Autodesk Inventor part; units mm, degrees
ref_plane "YZ Plane" through (0, 0, 0) normal (1, 0, 0) x (0, 1, 0)
ref_plane "XZ Plane" through (0, 0, 0) normal (0, 1, 0) x (-1, 0, 0)
ref_plane "XY Plane" through (0, 0, 0) normal (0, 0, 1) x (1, 0, 0)
sketch "Sketch1" plane through (0, 0, 0) normal (0, 0, 1) x (1, 0, 0)
  circle A0 centre (0, 0) radius 6.35
  dimension "d0" = 12.7
extrude "Extrusion1" add sketch "Sketch1" along normal blind 203.2
sketch "Sketch5" plane through (0, 0, 0) normal (0, 1, 0) x (-1, 0, 0)
  line L0 (0, 1.524) -> (-1.27, 1.524)
  line L1 (-6.35, 0) -> (6.35, 0)
  line L2 (-1.27, 0) -> (1.27, 0)
  line L3 (1.27, 1.524) -> (0, 1.524)
  line L4 (1.27, 1.524) -> (6.35, 1.524)
  line L5 (6.35, 0) -> (6.35, 203.2)
  line L6 (6.35, 1.524) -> (-6.35, 1.524)
  line L7 (-6.35, 1.524) -> (-6.35, 0)
  line L8 (-6.35, 0) -> (6.35, 0)
  line L9 (6.35, 0) -> (6.35, 1.524)
  line L10 (6.35, 203.2) -> (-6.35, 203.2)
  line L11 (-6.35, 203.2) -> (6.35, 203.2)
  line L12 (6.35, 203.2) -> (6.35, 201.676)
  line L13 (6.35, 201.676) -> (-6.35, 201.676)
  line L14 (-6.35, 201.676) -> (-6.35, 203.2)
  point P0 (0, 0)
  dimension "d20" = 1.524
  dimension "d21" = 1.27
  dimension "d26" = 12.7
  dimension "d27" = 1.524
sketch "Sketch7" plane through (0, 0, 0) normal (1, 0, 0) x (0, 1, 0)
  line L0 (0, 0) -> (0, 50.8)
  circle A0 centre (0, 50.8) radius 1.27
  line L1 (0, 50.8) -> (0, 101.6)
  circle A1 centre (0, 101.6) radius 1.27
  line L2 (0, 101.6) -> (0, 152.4)
  circle A2 centre (0, 152.4) radius 1.27
  dimension "d42" = 50.8
  dimension "d43" = 2.54
  dimension "d44" = 50.8
  dimension "d45" = 2.54
  dimension "d46" = 50.8
  dimension "d47" = 2.54
extrude "Extrusion8" cut sketch "Sketch7" along normal mid plane 25.4
extrude "Extrusion9" cut sketch "Sketch5" along normal mid plane 25.4 contours L13 L14 L10 L5
properties part number "Straw"
Work out the finished part from the listing and answer in its coordinate system (mm). Coordinates: 2 decimals unless noted, no trailing zeros. Write each loop counter-clockwise with the first axis right and the second up, starting at its lowest first coordinate (ties: lowest second). Pieces come first, ordered by that corner, then holes. Notation, with made-up numbers: M -38,70 L -3,70 A23 cw -3,94 Z; hole C 70.5,-10 d8. An arc over 180 degrees is marked long. Write item = value, one per line.
1. The part is cut by section B-B (z = 173). Determine the outline of the cut face in (x, y), then the cut area to 3 significant figures.
Solution:
outline = C 0,0 d12.7
area = 127 mm2
2. The part is cut by section A-A (x = 1). Determine the outline of the cut face in (y, z).
Solution:
outline = M -6.27,0 L 6.27,0 L 6.27,201.68 L -6.27,201.68 Z; hole C 0,50.8 d2.54; hole C 0,101.6 d2.54; hole C 0,152.4 d2.54
3. Straight lines are drawn through the part: line 1 (Z direction, x = -1.75, y = 0); line 2 (Z direction, x = -5.5, y = 0.75); line 3 (X direction, y = 0.25, z = 37). For each, find the intervals that lie inside material, in ascending order. Write a range as from..to.
Solution:
line_1 = 0..49.53, 52.07..100.33, 102.87..151.13, 153.67..201.68
line_2 = 0..49.78, 51.82..100.58, 102.62..151.38, 153.42..201.68
line_3 = -6.35..6.35
4. Flat-ended cylindrical pins translate along their axes: pin 1 (3 mm diameter, centred on y = -4.5, z = 131, fed in from +X); pin 2 (1.5 mm diameter, centred on y = 3.5, z = 98.5, fed in from +X). Find the tip coordinate at first contact, or state that the pin passes through.
Solution:
pin_1 = 5.6
pin_2 = 5.72
